```python
from build123d import *

# Parameters (mm, degrees)
SKETCH_1_W              = 40.7
SKETCH_1_H              = 35
EXTRUDE_BOSS_DEPTH      = 10.25
EXTRUDE_2_DEPTH         = 2
EXTRUDE_CUT_DEPTH       = 18.5
CROQUIS10_R             = 7
SALIENTE_EXTRUIR5_DEPTH = 0.75
CROQUIS11_R             = 5.5
SALIENTE_EXTRUIR6_DEPTH = 1
CROQUIS12_R             = 3
SALIENTE_EXTRUIR7_DEPTH = 10
CHAFL_N2_SIZE           = 0.5
SKETCH1_W               = 7
SKETCH1_H               = 20.5
BOSS_EXTRUDE1_DEPTH     = 3


with BuildPart() as part:
    # Sketch 1 → Extrude Boss (new, symmetric)
    with BuildSketch(Plane.XY):
        Rectangle(SKETCH_1_W, SKETCH_1_H)
    extrude(amount=EXTRUDE_BOSS_DEPTH, both=True)

    # Sketch 3 → Extrude 2 (add)
    with BuildSketch(Plane(origin=(0, 17.5, 0), x_dir=(1, 0, 0), z_dir=(0, 1, 0))):
        with BuildLine():
            Line((10.1, 9.25), (-19.35, 9.25))
            Line((-19.35, 9.25), (-19.35, -9.25))
            Line((-19.35, -9.25), (10.1, -9.25))
            ThreePointArc((10.1, -9.25), (19.35, 0), (10.1, 9.25))
        make_face()
    extrude(amount=EXTRUDE_2_DEPTH)

    # Sketch 4 → Extrude Cut (cut)
    with BuildSketch(Plane.XY.offset(9.25)):
        Polygon((-19.35, 19.5), (-19.35, 18.5), (-15.35, 18.5), (-14.35, 19.5), align=None)
    extrude(amount=-EXTRUDE_CUT_DEPTH, mode=Mode.SUBTRACT)

    # Croquis10 → Saliente-Extruir5 (add)
    with BuildSketch(Plane(origin=(0, 19.5, 0), x_dir=(1, 0, 0), z_dir=(0, 1, 0))):
        with Locations(Location((10.1, 0, 0), (0, 0, 270))):
            Circle(CROQUIS10_R)
    extrude(amount=SALIENTE_EXTRUIR5_DEPTH)

    # Croquis11 → Saliente-Extruir6 (add)
    with BuildSketch(Plane(origin=(0, 20.25, 0), x_dir=(1, 0, 0), z_dir=(0, 1, 0))):
        with Locations(Location((10.1, 0, 0), (0, 0, 270))):
            Circle(CROQUIS11_R)
    extrude(amount=SALIENTE_EXTRUIR6_DEPTH)

    # Croquis12 → Saliente-Extruir7 (add)
    with BuildSketch(Plane(origin=(0, 21.25, 0), x_dir=(1, 0, 0), z_dir=(0, 1, 0))):
        with Locations(Location((10.1, 0, 0), (0, 0, 270))):
            Circle(CROQUIS12_R)
    extrude(amount=SALIENTE_EXTRUIR7_DEPTH)

    # Chaflán2
    chafl_n2_edges = [part.edges().sort_by_distance(p)[0] for p in [
        (19.35, 19.5, 0),
        (-2.125, 19.5, -9.25),
        (-2.125, 19.5, 9.25),
        (10.1, 31.25, -3),
    ]]
    chamfer(chafl_n2_edges, length=CHAFL_N2_SIZE)

    # Croquis13 → Cortar-Revolución1 (revolve, cut)
    with BuildSketch(Plane.XY, mode=Mode.PRIVATE) as cortar_revoluci_n1_sk:
        Polygon((7.1, 21.75), (7.1, 21.25), (7.6, 21.25), align=None)
    revolve(cortar_revoluci_n1_sk.sketch.rotate(Axis((10.1, 31.25, 0), (0, -1, 0)), 270), axis=Axis((10.1, 31.25, 0), (0, -1, 0)), mode=Mode.SUBTRACT)

    # Sketch1 → Boss-Extrude1 (add)
    with BuildSketch(Plane.XZ.offset(17.5)):
        with Locations((-23.85, 0)):
            Rectangle(SKETCH1_W, SKETCH1_H)
        with Locations((23.85, 0)):
            Rectangle(SKETCH1_W, SKETCH1_H)
    extrude(amount=-BOSS_EXTRUDE1_DEPTH)


solid = part.part
```
CAD build for the part. Positions are in the model's coordinates, mm. A direction names the side the tool comes from. Round coordinates to 2 decimals unless told otherwise and drop trailing zeros. Order: outer loops, then holes, each group sorted by start corner. A loop starts at its lowest first (then second) coordinate and runs counter-clockwise, first axis right, second up. Notation, with made-up numbers: (56, -21.5) - (93, -21.5) arc R25 cw to (93, -3.5) - close; hole circle Ø2 at (45, -15). An arc over 180 degrees is marked (long way). Use CSV: the item, a comma, the result in double quotes. Start each with the question number.
1) Saw through at C-C (y = -2.5). List the corners of the cut face in (x, z), and give its area (3 significant figures).
2) Pin check, flat tips, straight feed: pin 1 Ø3 at (x, z) = (-16.5, -1) entering from +Y; pin 2 Ø11 at (x, z) = (7, 0) entering from +Y; pin 3 Ø7.5 at (x, z) = (24, -4.5) entering from +Y; pin 4 Ø3 at (y, z) = (20, -2.5) entering from +X. Stop position of each tip, or through.
3) Saw through at B-B (x = -5). List the corners of the cut face in (y, z).
4) Saw through at D-D (x = 21). List the corners of the cut face in (y, z), and give its area (3 significant figures).
5) Tool access for faces 1 (the flat face through (20.35, 1, 0)), 2 (the flat face through (5, 20.25, 3)), 3 (the flat face through (13, 21.25, 0)): list every direction of +Z, -Z, +X, -X, +Y, -Y with a clear straight run to the whole face (end or side of a thin tool).
6) Wall check: L1, parallel to Y at x = -16.5, z = 9; L2, parallel to Y at x = 6.5, z = -5.5; L3, parallel to X at y = -11, z = 0. Give the ranges that are in metal, low to high. Write a range as [from, to].
Values follow:
1,outline,"(-20.35, -10.25) - (20.35, -10.25) - (20.35, 10.25) - (-20.35, 10.25) - close"
1,area,"834 mm2"
2,pin 1,"stops at y = 18.85"
2,pin 2,"stops at y = 31.25"
2,pin 3,"stops at y = 17.5"
2,pin 4,"stops at x = 19.25"
3,outline,"(-17.5, -10.25) - (17.5, -10.25) - (17.5, -9.25) - (19, -9.25) - (19.5, -8.75) - (19.5, 8.75) - (19, 9.25) - (17.5, 9.25) - (17.5, 10.25) - (-17.5, 10.25) - close"
4,outline,"(-17.5, -10.25) - (-14.5, -10.25) - (-14.5, 10.25) - (-17.5, 10.25) - close"
4,area,"61.5 mm2"
5,face 1,"+Z, -Z, +X, +Y"
5,face 2,"+Y"
5,face 3,"none"
6,L1,"y = [-17.5, 18.5]"
6,L2,"y = [-17.5, 20.25]"
6,L3,"x = [-20.35, 20.35]"
